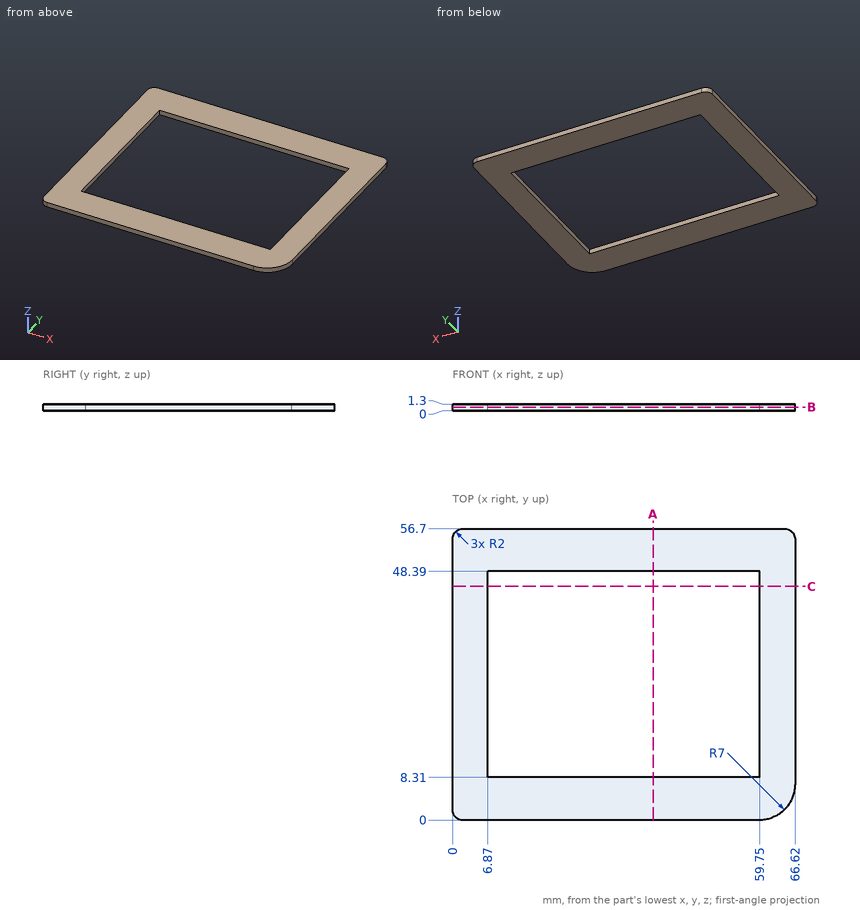
Verification items for this drawing (mm, ordinates from the low corner). Coordinates: 2 decimals unless noted, no trailing zeros. Write each loop counter-clockwise with the first axis right and the second up, starting at its lowest first coordinate (ties: lowest second). Pieces come first, ordered by that corner, then holes. Notation, with made-up numbers: M 61.25,89.25 L 80.25,89.25 A29 ccw 80.25,114.25 Z; hole C 78.25,-25 d11. An arc over 180 degrees is marked long. One line per item, written item: value. Start each with the question number.
(1) Sectioned sample at A-A, the plane x = 39. Enter the section's corners in (y, z).
(2) Sectioned sample at C-C, the plane y = 45.5. Enter the section's corners in (x, z), and give its area (3 significant figures).
(3) Depth check by flat-ended pin: pin 1 (3 mm diameter, centred on x = 57, y = 47, fed in from -Z). Enter the tip coordinate at first touch or a pass-through.
(4) Sectioned sample at B-B, the plane z = 0.7. Enter the section's corners in (x, y).
(5) Scan lines: line 1 along Y through (x, z) = (18, 0.15); line 2 along X through (y, z) = (44, 1.25); line 3 along X through (y, z) = (4.5, 0.55). Record each from-to range of solid material in increasing order. Write a range as [from, to].
Filled sheet:
1. outline: M 0,0 L 8.31,0 L 8.31,1.3 L 0,1.3 Z; M 48.39,0 L 56.7,0 L 56.7,1.3 L 48.39,1.3 Z
2. outline: M 0,0 L 6.87,0 L 6.87,1.3 L 0,1.3 Z; M 59.75,0 L 66.62,0 L 66.62,1.3 L 59.75,1.3 Z
2. area: 17.9 mm²
3. pin 1: z = 0
4. outline: M 0,2 A2 ccw 2,0 L 59.62,0 A7 ccw 66.62,7 L 66.62,54.7 A2 ccw 64.62,56.7 L 2,56.7 A2 ccw 0,54.7 Z; hole M 6.87,8.31 L 59.75,8.31 L 59.75,48.39 L 6.87,48.39 Z
5. line 1: [0, 8.31], [48.39, 56.7]
5. line 2: [0, 6.87], [59.75, 66.62]
5. line 3: [0, 66.16]
